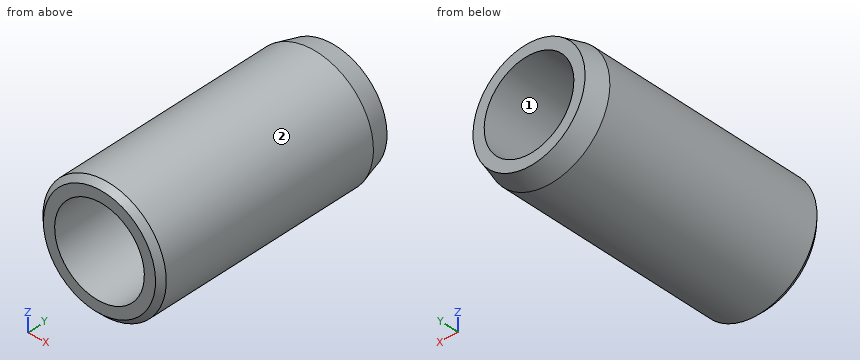
```python
from build123d import *

# Parameters (mm, degrees)
SKETCH1_R           = 22
SKETCH1_R_2         = 16
BOSS_EXTRUDE1_DEPTH = 90
CHAMFER1_SIZE       = 2
CHAMFER1_SIZE2      = 7.464101615
CHAMFER2_SIZE       = 2


with BuildPart() as part:
    # Sketch1 → Boss-Extrude1 (new body)
    with BuildSketch(Plane(origin=(0, 0, 0), x_dir=(1, 0, 0), z_dir=(0, 1, 0))):
        with Locations(Location((0, 0, 0), (0, 0, 270))):
            Circle(SKETCH1_R)
        with Locations(Location((0, 0, 0), (0, 0, 270))):
            Circle(SKETCH1_R_2, mode=Mode.SUBTRACT)
    extrude(amount=-BOSS_EXTRUDE1_DEPTH)

    # Chamfer1
    chamfer1_edges = [part.edges().sort_by_distance(p)[0] for p in [
        (0, 0, -22),
    ]]
    chamfer1_side = [part.faces().sort_by_distance(p)[0] for p in [
        (0, 0, -21.377746033),
    ]]
    chamfer(chamfer1_edges, length=CHAMFER1_SIZE, length2=CHAMFER1_SIZE2, reference=chamfer1_side[0])

    # Chamfer2
    chamfer2_edges = [part.edges().sort_by_distance(p)[0] for p in [
        (0, -90, -22),
    ]]
    chamfer(chamfer2_edges, length=CHAMFER2_SIZE)


solid = part.part
```
Could you check a few things on this model? Use its own coordinates, in mm. Face numbers are marked on the shaded views. Round coordinates to 2 decimals unless told otherwise and drop trailing zeros. Loops run counter-clockwise (first coordinate to the right, second up) from the corner with the lowest first, then second, coordinate; pieces in that order, holes last. Notation, with made-up numbers: (-17.5, 19.25) - (-7.5, 19.25) arc R12 cw to (-7.5, 40.25) - close; hole circle Ø11 at (5, 36). An arc over 180 degrees is marked (long way). Answer in a Markdown table with one row per item. Add a question column.
(1) If we section it at C-C (y = -32.5): Please give me the cut outline in (x, z).
(2) If we section it at A-A (x = 0): Please give me the cut outline in (y, z).
(3) If we mould it in two halves opening along X, with no side actions, what happens to the marked faces 1 and 2? For each: pulls with the +X half, pulls with the -X half, needs draft (parallel to the pull), parting line crosses it, or undercut.
(4) I'm going to push flat-ended pins straight in: pin 1 (6 mm diameter, centred on x = 7, y = -48, fed in from -Z); pin 2 (3 mm diameter, centred on x = 15, y = -63, fed in from +Z); pin 3 (1.5 mm diameter, centred on x = 3.5, y = -50, fed in from -Z). Where does each tip first touch, or does it pass through?
(5) If we section it at B-B (z = 0): Please give me the cut outline in (x, y).
(6) I need wall thicknesses on line 1 along X through (y, z) = (-44, 0); line 2 along Z through (x, y) = (-0.5, -32); line 3 along Z through (x, y) = (6, -69). Which ranges of each line are inside material? Lowest first, please.
Model answer:
| question | item | result |
|---|---|---|
| 1 | outline | circle Ø44 at (0, 0); hole circle Ø32 at (0, 0) |
| 2 | outline | (-90, -20) - (-88, -22) - (-7.46, -22) - (0, -20) - (0, -16) - (-90, -16) - close; (-90, 16) - (0, 16) - (0, 20) - (-7.46, 22) - (-88, 22) - (-90, 20) - close |
| 3 | face 1 | undercut |
| 3 | face 2 | parting line crosses it |
| 4 | pin 1 | stops at z = -21.63 |
| 4 | pin 2 | stops at z = 17.37 |
| 4 | pin 3 | stops at z = -21.83 |
| 5 | outline | (-22, -88) - (-20, -90) - (-16, -90) - (-16, 0) - (-20, 0) - (-22, -7.46) - close; (16, -90) - (20, -90) - (22, -88) - (22, -7.46) - (20, 0) - (16, 0) - close |
| 6 | line 1 | x = -22 to -16, 16 to 22 |
| 6 | line 2 | z = -21.99 to -15.99, 15.99 to 21.99 |
| 6 | line 3 | z = -21.17 to -14.83, 14.83 to 21.17 |
